Verification items for the finished model (mm, model axes). Face numbers are marked on the shaded views. A direction names the side the tool comes from. Coordinates: 2 decimals unless noted, no trailing zeros. Write each loop counter-clockwise with the first axis right and the second up, starting at its lowest first coordinate (ties: lowest second). Pieces come first, ordered by that corner, then holes. Notation, with made-up numbers: (-22, 3.5) - (-11, 3.5) arc R11 cw to (-11, 24.5) - close; hole circle Ø1 at (11.25, 57). An arc over 180 degrees is marked (long way). Use one line per item in the form item = value. Start each with the question number.
(1) Sectioned sample at D-D (x = -80). Record the cut outline in (y, z), and give its area (3 significant figures).
(2) Gauge pin test, flat ends, axial feed: pin 1 Ø5 at (y, z) = (-27, 25) entering from +X; pin 2 Ø8 at (x, y) = (56, -46) entering from -Z; pin 3 Ø6 at (x, y) = (40.5, -82) entering from +Z; pin 4 Ø8 at (y, z) = (-40, 16.5) entering from -X. Record the tip position at first contact, or that the pin passes through.
(3) Material ranges on line 1 (Z direction, x = -23.5, y = -115); line 2 (X direction, y = 10.5, z = 44.5); line 3 (Z direction, x = 3.5, y = -49.5), recorded low to high. Write a range as [from, to].
(4) Sectioned sample at B-B (y = -25). Record the cut outline in (x, z), and give its area (3 significant figures).
(5) Sectioned sample at A-A (z = 39). Record the cut outline in (x, y), and give its area (3 significant figures).
(6) Tool access check on the marked faces 1 and 2. Record the directions out of +Z, -Z, +X, -X, +Y, -Y that give a thin tool (end or side, any length) a straight path to the whole face; none if there is none.
(7) Sectioned sample at C-C (x = -2.5). Record the cut outline in (y, z), and give its area (3 significant figures).
from build123d import *

# Parameters (mm, degrees)
F1_W     = 99.3970142677
F1_H     = 300
F1_R     = 8.75
F2_DEPTH = 12
F4_DEPTH = 6
F6_D     = 22
F8_R     = 50
F9_R     = 15


with BuildPart() as f2:
    # F1 (on face) → F2 (new body)
    with BuildSketch(Plane.XY):
        with Locations((-49.6985071339, 12.607654488)):
            Rectangle(F1_W, F1_H)
        with Locations((-48.6155549591, -77.3908188095)):
            Circle(F1_R, mode=Mode.SUBTRACT)
        with Locations((-49.0062846134, 22.6084178392)):
            Circle(F1_R, mode=Mode.SUBTRACT)
        with Locations((-49.3970142677, 122.607654488)):
            Circle(F1_R, mode=Mode.SUBTRACT)
    extrude(amount=F2_DEPTH)

    # F3 (on Right) → F4 (join)
    with BuildSketch(Plane.YZ):
        Polygon((-62.392345512, 12.4983141385), (-62.392345512, 0), (87.607654488, 0), (87.607654488, 13.4828369309), (37.607654488, 56.2372539129), (-12.392345512, 56.2372539129), align=None)
    extrude(amount=-F4_DEPTH)

    # F6 (through all)
    with Locations(Plane.YZ):
        with Locations((12.607654488, 33.2372539129)):
            Hole(F6_D / 2)

    # F7: F2 across face


with BuildPart() as f2_1:
    add(f2.part)
    add(f2.part.mirror(Plane(origin=(0, 12.7942838573, 18.839447443), x_dir=(0, 1, 0), z_dir=(1, 0, 0))))

    # F8
    f8_edges = [f2_1.edges().sort_by_distance(p)[0] for p in [
        (-99.397014, 162.607654, 6),
        (99.397014, 162.607654, 6),
        (99.397014, -137.392346, 6),
        (-99.397014, -137.392346, 6),
    ]]
    fillet(f8_edges, radius=F8_R)

    # F9
    f9_edges = [f2_1.edges().sort_by_distance(p)[0] for p in [
        (0, 37.607654, 56.237254),
        (0, -12.392346, 56.237254),
    ]]
    fillet(f9_edges, radius=F9_R)


solid = f2_1.part
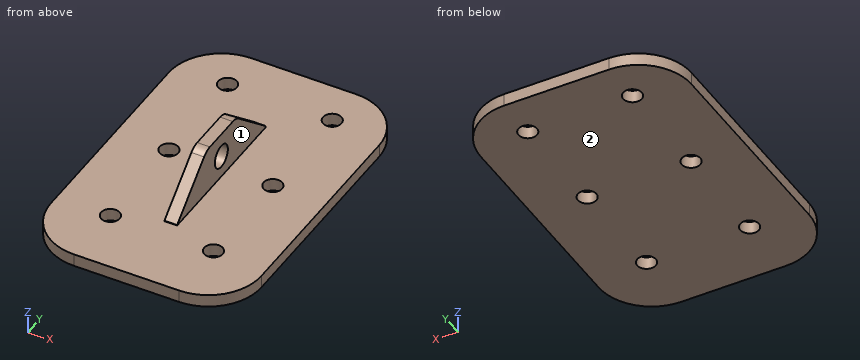
Answers below:
q1.outline = (-126.93, 0) - (152.15, 0) - (152.15, 12) - (-126.93, 12) - close
q1.area = 3,350 mm2
q2.pin_1 = 6
q2.pin_2 = 0
q2.pin_3 = 12
q2.pin_4 = -6
q3.line_1 = [0, 12]
q3.line_2 = [-6, 6]
q3.line_3 = [0, 23.78]
q4.outline = (-99.4, 0) - (99.4, 0) - (99.4, 12) - (6, 12) - (6, 45.21) - (-6, 45.21) - (-6, 12) - (-99.4, 12) - close
q4.area = 2,780 mm2
q5.outline = (-6, -32.1) - (6, -32.1) - (6, 3.24) - (-6, 3.24) - close; (-6, 21.98) - (6, 21.98) - (6, 57.77) - (-6, 57.77) - close
q5.area = 853 mm2
q6.face_1 = +Z, +X, +Y, -Y
q6.face_2 = -Z, +X, -X, +Y, -Y
q7.outline = (-137.39, 0) - (162.61, 0) - (162.61, 12) - (87.61, 12) - (87.61, 13.48) - (41.82, 52.64) arc R15 ccw to (32.07, 56.24) - (-6.76, 56.24) arc R15 ccw to (-16.63, 52.53) - (-62.39, 12.5) - (-62.39, 12) - (-137.39, 12) - close; hole circle Ø22 at (12.61, 33.24)
q7.area = 7,690 mm2
